from build123d import *

# Parameters (mm, degrees)
F0_W     = 32.402042
F0_H     = 68.217468
F0_R     = 12.5
F1_DEPTH = 5


with BuildPart() as f1:
    # F0 (on Front) → F1 (new body, symmetric)
    with BuildSketch(Plane.XZ):
        with Locations((0, 17.5768)):
            Rectangle(F0_W, F0_H)
        Circle(F0_R, mode=Mode.SUBTRACT)
        with Locations((0, 35.1536)):
            Circle(F0_R, mode=Mode.SUBTRACT)
    extrude(amount=F1_DEPTH, both=True)


solid = f1.part
Geometry: final body of the model. Coordinates: model frame, mm. Coordinates: 2 decimals unless noted, no trailing zeros. Loops run counter-clockwise (first coordinate to the right, second up) from the corner with the lowest first, then second, coordinate; pieces in that order, holes last. Notation, with made-up numbers: (1.5, 9) - (52.5, 9) arc R21 cw to (52.5, 21) - close; hole circle Ø7 at (88.25, 81). An arc over 180 degrees is marked (long way). Put each result on its own line as item: value. Start each with the question number.
Q1. Line query: line 1 (Z direction, x = 0, y = 0.5); line 2 (Z direction, x = -10, y = -2.25); line 3 (X direction, y = 1.75, z = 36). Output: solid intervals per line, ascending.
Q2. Cut plane A-A, the plane x = 0. Return loops of the section in (y, z), and give its area (3 significant figures).
Q3. Cut plane C-C, the plane y = 2.5. Return loops of the section in (x, z), and give its area (3 significant figures).
Q4. Cut plane D-D, the plane x = 7.5. Return loops of the section in (y, z), and give its area (3 significant figures).
Q5. Pin query (flat end, axial travel): pin 1 Ø6 at (x, z) = (-1, 43.5) entering from -Y. Return the tip coordinate at first contact, or that it passes through.
Q6. Pull-direction query (X, two-part tool) for faces 1 (the flat face through (0, 5, 18)), 2 (the flat face through (-16.201, 0, 17)), 3 (the cylindrical face through (11.923, 0.07, 3.755)), 4 (the cylindrical face through (11.923, 0.07, 38.908)); classes: released by +X, released by -X, zero draft, split by the parting line, or undercut.
Q7. Cut plane B-B, the plane z = 0. Return loops of the section in (x, y), and give its area (3 significant figures).
Filled sheet:
1. line 1: -16.53 to -12.5, 12.5 to 22.65, 47.65 to 51.69
1. line 2: -16.53 to -7.5, 7.5 to 27.65, 42.65 to 51.69
1. line 3: -16.2 to -12.47, 12.47 to 16.2
2. outline: (-5, -16.53) - (5, -16.53) - (5, -12.5) - (-5, -12.5) - close; (-5, 12.5) - (5, 12.5) - (5, 22.65) - (-5, 22.65) - close; (-5, 47.65) - (5, 47.65) - (5, 51.69) - (-5, 51.69) - close
2. area: 182 mm²
3. outline: (-16.2, -16.53) - (16.2, -16.53) - (16.2, 51.69) - (-16.2, 51.69) - close; hole circle Ø25 at (0, 0); hole circle Ø25 at (0, 35.15)
3. area: 1,230 mm²
4. outline: (-5, -16.53) - (5, -16.53) - (5, -10) - (-5, -10) - close; (-5, 10) - (5, 10) - (5, 25.15) - (-5, 25.15) - close; (-5, 45.15) - (5, 45.15) - (5, 51.69) - (-5, 51.69) - close
4. area: 282 mm²
5. pin 1: through
6. face 1: zero draft
6. face 2: released by -X
6. face 3: undercut
6. face 4: undercut
7. outline: (-16.2, -5) - (-12.5, -5) - (-12.5, 5) - (-16.2, 5) - close; (12.5, -5) - (16.2, -5) - (16.2, 5) - (12.5, 5) - close
7. area: 74.0 mm²
